from build123d import *
from OCP.BRepFilletAPI import BRepFilletAPI_MakeChamfer

# Parameters (mm, degrees)
BOSS_EXTRUDE1_DEPTH  = 2.286
BOSS_EXTRUDE2_DEPTH  = 0.254
BOSS_EXTRUDE3_DEPTH  = 0.254
BOSS_EXTRUDE4_DEPTH  = 0.254
BOSS_EXTRUDE5_DEPTH  = 0.254
BOSS_EXTRUDE6_DEPTH  = 0.254
BOSS_EXTRUDE7_DEPTH  = 0.254
BOSS_EXTRUDE8_DEPTH  = 0.254
SKETCH9_W            = 0.65
SKETCH9_H            = 0.65
BOSS_EXTRUDE9_DEPTH  = 3.302
SKETCH10_W           = 0.65
SKETCH10_H           = 0.65
BOSS_EXTRUDE10_DEPTH = 6.35
SKETCH11_W           = 0.65
SKETCH11_H           = 0.65
BOSS_EXTRUDE11_DEPTH = 3.302
SKETCH12_W           = 0.65
SKETCH12_H           = 0.65
BOSS_EXTRUDE12_DEPTH = 6.35
SKETCH13_W           = 0.65
SKETCH13_H           = 0.65
BOSS_EXTRUDE13_DEPTH = 3.302
SKETCH14_W           = 0.65
SKETCH14_H           = 0.65
BOSS_EXTRUDE14_DEPTH = 6.35
SKETCH15_W           = 0.65
SKETCH15_H           = 0.65
BOSS_EXTRUDE15_DEPTH = 3.302
SKETCH16_W           = 0.65
SKETCH16_H           = 0.65
BOSS_EXTRUDE16_DEPTH = 6.35
SKETCH17_W           = 0.65
SKETCH17_H           = 0.65
BOSS_EXTRUDE17_DEPTH = 3.302
SKETCH18_W           = 0.65
SKETCH18_H           = 0.65
BOSS_EXTRUDE18_DEPTH = 6.35
SKETCH19_W           = 0.65
SKETCH19_H           = 0.65
BOSS_EXTRUDE19_DEPTH = 3.302
SKETCH20_W           = 0.65
SKETCH20_H           = 0.65
BOSS_EXTRUDE20_DEPTH = 6.35
CHAMFER1_SIZE        = 0.2
CHAMFER1_SIZE2       = 0.4


with BuildPart() as part:
    # Sketch1 → Boss-Extrude1 (new body)
    with BuildSketch(Plane.XY.offset(2.54)):
        Polygon((13.97, -1.016), (13.97, 1.016), (13.716, 1.27), (11.684, 1.27), (11.43, 1.016), (11.176, 1.27), (9.144, 1.27), (8.89, 1.016), (8.636, 1.27), (6.604, 1.27), (6.35, 1.016), (6.096, 1.27), (4.064, 1.27), (3.81, 1.016), (3.556, 1.27), (1.524, 1.27), (1.27, 1.016), (1.016, 1.27), (-1.016, 1.27), (-1.27, 1.016), (-1.27, -1.016), (-1.016, -1.27), (1.016, -1.27), (1.27, -1.016), (1.524, -1.27), (3.556, -1.27), (3.81, -1.016), (4.064, -1.27), (6.096, -1.27), (6.35, -1.016), (6.604, -1.27), (8.636, -1.27), (8.89, -1.016), (9.144, -1.27), (11.176, -1.27), (11.43, -1.016), (11.684, -1.27), (13.716, -1.27), align=None)
    extrude(amount=-BOSS_EXTRUDE1_DEPTH)

    # Sketch2 → Boss-Extrude2 (add)
    with BuildSketch(Plane(origin=(0, 0, 0.254), x_dir=(-1, 0, 0), z_dir=(0, 0, -1))):
        Polygon((-6.604, -1.27), (-6.604, 1.27), (-6.35, 1.016), (-6.096, 1.27), (-6.096, -1.27), (-6.35, -1.016), align=None)
    extrude(amount=BOSS_EXTRUDE2_DEPTH)

    # Sketch3 → Boss-Extrude3 (add)
    with BuildSketch(Plane(origin=(0, 0, 0.254), x_dir=(-1, 0, 0), z_dir=(0, 0, -1))):
        Polygon((-9.144, -1.27), (-9.144, 1.27), (-8.89, 1.016), (-8.636, 1.27), (-8.636, -1.27), (-8.89, -1.016), align=None)
    extrude(amount=BOSS_EXTRUDE3_DEPTH)

    # Sketch4 → Boss-Extrude4 (add)
    with BuildSketch(Plane(origin=(0, 0, 0.254), x_dir=(-1, 0, 0), z_dir=(0, 0, -1))):
        Polygon((-11.684, -1.27), (-11.684, 1.27), (-11.43, 1.016), (-11.176, 1.27), (-11.176, -1.27), (-11.43, -1.016), align=None)
    extrude(amount=BOSS_EXTRUDE4_DEPTH)

    # Sketch5 → Boss-Extrude5 (add)
    with BuildSketch(Plane(origin=(0, 0, 0.254), x_dir=(-1, 0, 0), z_dir=(0, 0, -1))):
        Polygon((-4.064, -1.27), (-4.064, 1.27), (-3.81, 1.016), (-3.556, 1.27), (-3.556, -1.27), (-3.81, -1.016), align=None)
    extrude(amount=BOSS_EXTRUDE5_DEPTH)

    # Sketch6 → Boss-Extrude6 (add)
    with BuildSketch(Plane(origin=(0, 0, 0.254), x_dir=(-1, 0, 0), z_dir=(0, 0, -1))):
        Polygon((-1.524, -1.27), (-1.524, 1.27), (-1.27, 1.016), (-1.016, 1.27), (-1.016, -1.27), (-1.27, -1.016), align=None)
    extrude(amount=BOSS_EXTRUDE6_DEPTH)

    # Sketch7 → Boss-Extrude7 (add)
    with BuildSketch(Plane(origin=(0, 0, 0.254), x_dir=(-1, 0, 0), z_dir=(0, 0, -1))):
        Polygon((1.016, -1.27), (1.016, 1.27), (1.27, 1.016), (1.27, -1.016), align=None)
    extrude(amount=BOSS_EXTRUDE7_DEPTH)

    # Sketch8 → Boss-Extrude8 (add)
    with BuildSketch(Plane(origin=(0, 0, 0.254), x_dir=(-1, 0, 0), z_dir=(0, 0, -1))):
        Polygon((-13.97, -1.016), (-13.97, 1.016), (-13.716, 1.27), (-13.716, -1.27), align=None)
    extrude(amount=BOSS_EXTRUDE8_DEPTH)

    # Sketch9 → Boss-Extrude9 (add)
    with BuildSketch(Plane(origin=(0, 0, 0.254), x_dir=(-1, 0, 0), z_dir=(0, 0, -1))):
        Rectangle(SKETCH9_W, SKETCH9_H)
    extrude(amount=BOSS_EXTRUDE9_DEPTH)

    # Sketch10 → Boss-Extrude10 (add)
    with BuildSketch(Plane.XY.offset(2.54)):
        Rectangle(SKETCH10_W, SKETCH10_H)
    extrude(amount=BOSS_EXTRUDE10_DEPTH)

    # Sketch11 → Boss-Extrude11 (add)
    with BuildSketch(Plane(origin=(0, 0, 0.254), x_dir=(-1, 0, 0), z_dir=(0, 0, -1))):
        with Locations((-12.7, 0)):
            Rectangle(SKETCH11_W, SKETCH11_H)
    extrude(amount=BOSS_EXTRUDE11_DEPTH)

    # Sketch12 → Boss-Extrude12 (add)
    with BuildSketch(Plane.XY.offset(2.54)):
        with Locations((12.7, 0)):
            Rectangle(SKETCH12_W, SKETCH12_H)
    extrude(amount=BOSS_EXTRUDE12_DEPTH)

    # Sketch13 → Boss-Extrude13 (add)
    with BuildSketch(Plane(origin=(0, 0, 0.254), x_dir=(-1, 0, 0), z_dir=(0, 0, -1))):
        with Locations((-10.16, 0)):
            Rectangle(SKETCH13_W, SKETCH13_H)
    extrude(amount=BOSS_EXTRUDE13_DEPTH)

    # Sketch14 → Boss-Extrude14 (add)
    with BuildSketch(Plane.XY.offset(2.54)):
        with Locations((10.16, 0)):
            Rectangle(SKETCH14_W, SKETCH14_H)
    extrude(amount=BOSS_EXTRUDE14_DEPTH)

    # Sketch15 → Boss-Extrude15 (add)
    with BuildSketch(Plane(origin=(0, 0, 0.254), x_dir=(-1, 0, 0), z_dir=(0, 0, -1))):
        with Locations((-7.62, 0)):
            Rectangle(SKETCH15_W, SKETCH15_H)
    extrude(amount=BOSS_EXTRUDE15_DEPTH)

    # Sketch16 → Boss-Extrude16 (add)
    with BuildSketch(Plane.XY.offset(2.54)):
        with Locations((7.62, 0)):
            Rectangle(SKETCH16_W, SKETCH16_H)
    extrude(amount=BOSS_EXTRUDE16_DEPTH)

    # Sketch17 → Boss-Extrude17 (add)
    with BuildSketch(Plane(origin=(0, 0, 0.254), x_dir=(-1, 0, 0), z_dir=(0, 0, -1))):
        with Locations((-5.08, 0)):
            Rectangle(SKETCH17_W, SKETCH17_H)
    extrude(amount=BOSS_EXTRUDE17_DEPTH)

    # Sketch18 → Boss-Extrude18 (add)
    with BuildSketch(Plane.XY.offset(2.54)):
        with Locations((5.08, 0)):
            Rectangle(SKETCH18_W, SKETCH18_H)
    extrude(amount=BOSS_EXTRUDE18_DEPTH)

    # Sketch19 → Boss-Extrude19 (add)
    with BuildSketch(Plane(origin=(0, 0, 0.254), x_dir=(-1, 0, 0), z_dir=(0, 0, -1))):
        with Locations((-2.54, 0)):
            Rectangle(SKETCH19_W, SKETCH19_H)
    extrude(amount=BOSS_EXTRUDE19_DEPTH)

    # Sketch20 → Boss-Extrude20 (add)
    with BuildSketch(Plane.XY.offset(2.54)):
        with Locations((2.54, 0)):
            Rectangle(SKETCH20_W, SKETCH20_H)
    extrude(amount=BOSS_EXTRUDE20_DEPTH)

    # Chamfer1: one chamfer whose edges measure the first distance from different faces: ONE call of the kernel's chamfer builder (chamfer() names one face for all edges)
    chamfer1_edges_1 = [part.edges().sort_by_distance(p)[0] for p in [
        (0, 0.325, -3.048),
        (0.325, 0, -3.048),
        (0, -0.325, -3.048),
        (-0.325, 0, -3.048),
    ]]
    chamfer1_side_1 = [part.faces().sort_by_distance(p)[0] for p in [
        (0, 0, -3.048),
    ]]
    chamfer1_edges_2 = [part.edges().sort_by_distance(p)[0] for p in [
        (0, -0.325, 8.89),
        (0.325, 0, 8.89),
        (0, 0.325, 8.89),
        (-0.325, 0, 8.89),
    ]]
    chamfer1_side_2 = [part.faces().sort_by_distance(p)[0] for p in [
        (0, 0, 8.89),
    ]]
    chamfer1_edges_3 = [part.edges().sort_by_distance(p)[0] for p in [
        (12.375, 0, -3.048),
        (12.7, 0.325, -3.048),
        (13.025, 0, -3.048),
        (12.7, -0.325, -3.048),
    ]]
    chamfer1_side_3 = [part.faces().sort_by_distance(p)[0] for p in [
        (12.7, 0, -3.048),
    ]]
    chamfer1_edges_4 = [part.edges().sort_by_distance(p)[0] for p in [
        (12.7, -0.325, 8.89),
        (13.025, 0, 8.89),
        (12.7, 0.325, 8.89),
        (12.375, 0, 8.89),
    ]]
    chamfer1_side_4 = [part.faces().sort_by_distance(p)[0] for p in [
        (12.7, 0, 8.89),
    ]]
    chamfer1_edges_5 = [part.edges().sort_by_distance(p)[0] for p in [
        (9.835, 0, -3.048),
        (10.16, 0.325, -3.048),
        (10.485, 0, -3.048),
        (10.16, -0.325, -3.048),
    ]]
    chamfer1_side_5 = [part.faces().sort_by_distance(p)[0] for p in [
        (10.16, 0, -3.048),
    ]]
    chamfer1_edges_6 = [part.edges().sort_by_distance(p)[0] for p in [
        (10.16, -0.325, 8.89),
        (10.485, 0, 8.89),
        (10.16, 0.325, 8.89),
        (9.835, 0, 8.89),
    ]]
    chamfer1_side_6 = [part.faces().sort_by_distance(p)[0] for p in [
        (10.16, 0, 8.89),
    ]]
    chamfer1_edges_7 = [part.edges().sort_by_distance(p)[0] for p in [
        (7.945, 0, -3.048),
        (7.62, -0.325, -3.048),
        (7.295, 0, -3.048),
        (7.62, 0.325, -3.048),
    ]]
    chamfer1_side_7 = [part.faces().sort_by_distance(p)[0] for p in [
        (7.62, 0, -3.048),
    ]]
    chamfer1_edges_8 = [part.edges().sort_by_distance(p)[0] for p in [
        (7.62, 0.325, 8.89),
        (7.295, 0, 8.89),
        (7.62, -0.325, 8.89),
        (7.945, 0, 8.89),
    ]]
    chamfer1_side_8 = [part.faces().sort_by_distance(p)[0] for p in [
        (7.62, 0, 8.89),
    ]]
    chamfer1_edges_9 = [part.edges().sort_by_distance(p)[0] for p in [
        (5.405, 0, -3.048),
        (5.08, -0.325, -3.048),
        (4.755, 0, -3.048),
        (5.08, 0.325, -3.048),
    ]]
    chamfer1_side_9 = [part.faces().sort_by_distance(p)[0] for p in [
        (5.08, 0, -3.048),
    ]]
    chamfer1_edges_10 = [part.edges().sort_by_distance(p)[0] for p in [
        (5.08, 0.325, 8.89),
        (4.755, 0, 8.89),
        (5.08, -0.325, 8.89),
        (5.405, 0, 8.89),
    ]]
    chamfer1_side_10 = [part.faces().sort_by_distance(p)[0] for p in [
        (5.08, 0, 8.89),
    ]]
    chamfer1_edges_11 = [part.edges().sort_by_distance(p)[0] for p in [
        (2.865, 0, -3.048),
        (2.54, -0.325, -3.048),
        (2.215, 0, -3.048),
        (2.54, 0.325, -3.048),
    ]]
    chamfer1_side_11 = [part.faces().sort_by_distance(p)[0] for p in [
        (2.54, 0, -3.048),
    ]]
    chamfer1_edges_12 = [part.edges().sort_by_distance(p)[0] for p in [
        (2.54, 0.325, 8.89),
        (2.215, 0, 8.89),
        (2.54, -0.325, 8.89),
        (2.865, 0, 8.89),
    ]]
    chamfer1_side_12 = [part.faces().sort_by_distance(p)[0] for p in [
        (2.54, 0, 8.89),
    ]]
    chamfer1 = BRepFilletAPI_MakeChamfer(part.part.solid().wrapped)
    for e in chamfer1_edges_1:
        chamfer1.Add(CHAMFER1_SIZE, CHAMFER1_SIZE2, e.wrapped, chamfer1_side_1[0].wrapped)  # the first distance lies on this face
    for e in chamfer1_edges_2:
        chamfer1.Add(CHAMFER1_SIZE, CHAMFER1_SIZE2, e.wrapped, chamfer1_side_2[0].wrapped)  # the first distance lies on this face
    for e in chamfer1_edges_3:
        chamfer1.Add(CHAMFER1_SIZE, CHAMFER1_SIZE2, e.wrapped, chamfer1_side_3[0].wrapped)  # the first distance lies on this face
    for e in chamfer1_edges_4:
        chamfer1.Add(CHAMFER1_SIZE, CHAMFER1_SIZE2, e.wrapped, chamfer1_side_4[0].wrapped)  # the first distance lies on this face
    for e in chamfer1_edges_5:
        chamfer1.Add(CHAMFER1_SIZE, CHAMFER1_SIZE2, e.wrapped, chamfer1_side_5[0].wrapped)  # the first distance lies on this face
    for e in chamfer1_edges_6:
        chamfer1.Add(CHAMFER1_SIZE, CHAMFER1_SIZE2, e.wrapped, chamfer1_side_6[0].wrapped)  # the first distance lies on this face
    for e in chamfer1_edges_7:
        chamfer1.Add(CHAMFER1_SIZE, CHAMFER1_SIZE2, e.wrapped, chamfer1_side_7[0].wrapped)  # the first distance lies on this face
    for e in chamfer1_edges_8:
        chamfer1.Add(CHAMFER1_SIZE, CHAMFER1_SIZE2, e.wrapped, chamfer1_side_8[0].wrapped)  # the first distance lies on this face
    for e in chamfer1_edges_9:
        chamfer1.Add(CHAMFER1_SIZE, CHAMFER1_SIZE2, e.wrapped, chamfer1_side_9[0].wrapped)  # the first distance lies on this face
    for e in chamfer1_edges_10:
        chamfer1.Add(CHAMFER1_SIZE, CHAMFER1_SIZE2, e.wrapped, chamfer1_side_10[0].wrapped)  # the first distance lies on this face
    for e in chamfer1_edges_11:
        chamfer1.Add(CHAMFER1_SIZE, CHAMFER1_SIZE2, e.wrapped, chamfer1_side_11[0].wrapped)  # the first distance lies on this face
    for e in chamfer1_edges_12:
        chamfer1.Add(CHAMFER1_SIZE, CHAMFER1_SIZE2, e.wrapped, chamfer1_side_12[0].wrapped)  # the first distance lies on this face
    add(Compound.cast(chamfer1.Shape()), mode=Mode.REPLACE)


solid = part.part
Could you check a few things on this model? Use its own coordinates, in mm. Round coordinates to 2 decimals unless told otherwise and drop trailing zeros. Order: outer loops, then holes, each group sorted by start corner. A loop starts at its lowest first (then second) coordinate and runs counter-clockwise, first axis right, second up.
Q1. Please list where these lines run through material, in increasing order: probe 1 along X at (y, z) = (0.2, 3.75) (3 decimals); probe 2 along Z at (x, y) = (2.5, -0.65); probe 3 along Y at (x, z) = (12.75, -0.75) (3 decimals).
Geometry says:
probe 1: x = -0.325 to 0.325, 2.215 to 2.865, 4.755 to 5.405, 7.295 to 7.945, 9.835 to 10.485, 12.375 to 13.025
probe 2: z = 0.25 to 2.54
probe 3: y = -0.325 to 0.325
Q2. I'm going to push flat-ended pins straight in: P1, Ø0.7, axis at y = 0, z = 5.5, coming from the +X side (3 decimals); P2, Ø0.7, axis at x = 12.5, z = 6, coming from the -Y side (3 decimals); P3, Ø0.7, axis at x = 2.5, z = -1, coming from the +Y side (3 decimals). Where does each tip first touch, or does it pass through?
Geometry says:
P1: stops at x = 13.025
P2: stops at y = -0.325
P3: stops at y = 0.325
Q3. Imagine slicing it at B-B, the plane z = 6.75. List the corners of the cut face in (x, y) for me (3 decimals), then the cut area to 4 significant figures.
Geometry says:
outline: (-0.325, -0.325) - (0.325, -0.325) - (0.325, 0.325) - (-0.325, 0.325) - close; (2.215, -0.325) - (2.865, -0.325) - (2.865, 0.325) - (2.215, 0.325) - close; (4.755, -0.325) - (5.405, -0.325) - (5.405, 0.325) - (4.755, 0.325) - close; (7.295, -0.325) - (7.945, -0.325) - (7.945, 0.325) - (7.295, 0.325) - close; (9.835, -0.325) - (10.485, -0.325) - (10.485, 0.325) - (9.835, 0.325) - close; (12.375, -0.325) - (13.025, -0.325) - (13.025, 0.325) - (12.375, 0.325) - close
area: 2.535 mm2
Q4. Imagine slicing it at A-A, the plane y = 0.6. List the corners of the cut face in (x, z) for me.
Geometry says:
outline: (-1.27, 0) - (-1.02, 0) - (-1.02, 0.25) - (1.02, 0.25) - (1.02, 0) - (1.52, 0) - (1.52, 0.25) - (3.56, 0.25) - (3.56, 0) - (4.06, 0) - (4.06, 0.25) - (6.1, 0.25) - (6.1, 0) - (6.6, 0) - (6.6, 0.25) - (8.64, 0.25) - (8.64, 0) - (9.14, 0) - (9.14, 0.25) - (11.18, 0.25) - (11.18, 0) - (11.68, 0) - (11.68, 0.25) - (13.72, 0.25) - (13.72, 0) - (13.97, 0) - (13.97, 2.54) - (-1.27, 2.54) - close
Q5. Imagine slicing it at C-C, the plane x = 4.5. List the corners of the cut face in (y, z) for me.
Geometry says:
outline: (-1.27, 0.25) - (1.27, 0.25) - (1.27, 2.54) - (-1.27, 2.54) - close
